Input: part model. Units: mm. Frame: model coordinates. Coordinates: 2 decimals unless noted, no trailing zeros. Write each loop counter-clockwise with the first axis right and the second up, starting at its lowest first coordinate (ties: lowest second). Pieces come first, ordered by that corner, then holes.
1) Line query: L1, parallel to Y at x = 910.16, z = -0.5 (3 decimals); L2, parallel to X at y = 546.1, z = 2.25 (3 decimals); L3, parallel to Y at x = 1073, z = 4.75. Output: solid intervals per line, ascending.
2) Section query B-B (y = 546.1). Output: boundary loops of the cut face in (x, z) (3 decimals).
3) Section query A-A (x = 910.16). Output: boundary loops of the cut face in (y, z) (3 decimals).
4) Section query D-D (x = 792.5). Output: boundary loops of the cut face in (y, z), then the cut area to 3 significant figures.
5) Section query C-C (z = 3). Output: boundary loops of the cut face in (x, y) (3 decimals).
6) Pin query (flat end, axial travel): pin 1 Ø4 at (x, z) = (1046.5, -5) entering from -Y; pin 2 Ø21.5 at (x, y) = (910.16, 546.1) entering from -Z; pin 3 Ø4 at (y, z) = (334, 0) entering from -X. Return the tip coordinate at first contact, or that it passes through.
from build123d import *

# Parameters (mm, degrees)
BOSS_EXTRUDE1_DEPTH = 6.35
SKETCH3_W           = 203.2
SKETCH3_H           = 12.7
BOSS_EXTRUDE2_DEPTH = 76.2
CAVITY1_START       = -6.35
CAVITY1_OUTLINE_R   = 12.7
CAVITY1_DEPTH       = 12.7
MOVE_FACE_HOLE_BY   = 0.635
SLOT_FILLET_R       = 3.175


# Read off the part's stored shape, not the designer's step: Cavity1
with BuildPart() as part:
    # Sketch1 → Boss-Extrude1 (new, symmetric)
    with BuildSketch(Plane.XY):
        Polygon((732.36, 381), (785.7, 381), (1001.6, 381), (1087.96, 381), (1087.96, 685.8), (1001.6, 685.8), (785.7, 685.8), (732.36, 685.8), align=None)
    extrude(amount=BOSS_EXTRUDE1_DEPTH, both=True)

    # Sketch3 → Boss-Extrude2 (add)
    with BuildSketch(Plane.XZ.offset(-381)):
        with Locations((910.16, 0)):
            Rectangle(SKETCH3_W, SKETCH3_H)
    extrude(amount=BOSS_EXTRUDE2_DEPTH)

    # Cavity1 outline → Cavity1 (cut)
    with BuildSketch(Plane.XY.offset(CAVITY1_START)):
        with Locations((910.16, 546.1)):
            Circle(CAVITY1_OUTLINE_R)
    extrude(amount=CAVITY1_DEPTH, mode=Mode.SUBTRACT)

    # Move Face Hole: a curved face moved inward by 0.635
    add(Solid.thicken(part.faces().sort_by_distance((897.46, 546.1, 0))[0], -MOVE_FACE_HOLE_BY), mode=Mode.SUBTRACT)

    # Slot Fillet
    slot_fillet_edges = [part.edges().sort_by_distance(p)[0] for p in [
        (808.56, 381, 0),
        (1011.76, 381, 0),
    ]]
    fillet(slot_fillet_edges, radius=SLOT_FILLET_R)


solid = part.part
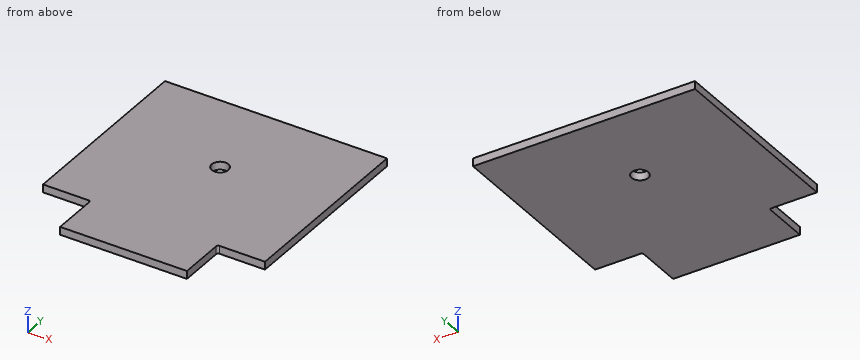
Answer:
1. L1: y = 304.8 to 532.765, 559.435 to 685.8
1. L2: x = 732.36 to 896.825, 923.495 to 1087.96
1. L3: y = 381 to 685.8
2. outline: (732.36, -6.35) - (896.825, -6.35) - (896.825, 6.35) - (732.36, 6.35) - close; (923.495, -6.35) - (1087.96, -6.35) - (1087.96, 6.35) - (923.495, 6.35) - close
3. outline: (304.8, -6.35) - (532.765, -6.35) - (532.765, 6.35) - (304.8, 6.35) - close; (559.435, -6.35) - (685.8, -6.35) - (685.8, 6.35) - (559.435, 6.35) - close
4. outline: (381, -6.35) - (685.8, -6.35) - (685.8, 6.35) - (381, 6.35) - close
4. area: 3,870 mm2
5. outline: (732.36, 381) - (805.385, 381) arc R3.175 cw to (808.56, 377.825) - (808.56, 304.8) - (1011.76, 304.8) - (1011.76, 377.825) arc R3.175 cw to (1014.935, 381) - (1087.96, 381) - (1087.96, 685.8) - (732.36, 685.8) - close; hole circle Ø26.67 at (910.16, 546.1)
6. pin 1: stops at y = 381
6. pin 2: passes through
6. pin 3: stops at x = 808.56
